Autodesk Inventor part; units mm, degrees
ref_plane "YZ Plane" through (0, 0, 0) normal (1, 0, 0) x (0, 1, 0)
ref_plane "XZ Plane" through (0, 0, 0) normal (0, 1, 0) x (-1, 0, 0)
ref_plane "XY Plane" through (0, 0, 0) normal (0, 0, 1) x (1, 0, 0)
sketch "스케치1" plane through (0, 0, 0) normal (1, 0, 0) x (0, 1, 0)
  circle A0 centre (0, 0) radius 55
  circle A1 centre (0, 0) radius 54
  dimension "d0" = 110
  dimension "d1" = 1
extrude "돌출1" add sketch "스케치1" along normal mid plane 36
sketch "스케치2" plane through (18, 0, 0) normal (1, 0, 0) x (0, 0, -1)
  circle A0 centre (0, 0) radius 55
  circle A1 centre (0, 0) radius 2
  dimension "d4" = 4
extrude "돌출2" add sketch "스케치2" against normal blind 1
sketch "스케치3" plane through (-18, 0, 0) normal (-1, 0, 0) x (0, 0, 1)
  circle A0 centre (0, 0) radius 2
  circle A1 centre (0, 0) radius 54
extrude "돌출3" add sketch "스케치3" against normal blind 1
sketch "스케치4" plane through (-18, 0, 0) normal (-1, 0, 0) x (0, 0, 1)
  circle A0 centre (0, 0) radius 14
  line L0 (0, 0) -> (14, 0)
  circle A1 centre (14, 0) radius 1.5
  dimension "d9" = 28
  dimension "d10" = 3
extrude "돌출4" cut sketch "스케치4" against normal blind 36 contours L0 A1 A0 | A0 A1 | A0 A1 L0 picked at (14.4441, -0.3905)
pattern_circular "원형 패턴1" count 4 over 360 about axis through (-18, 0, 0) along (1, 0, 0) of "돌출4"
fillet "모깎기1" radius 2 3 edges at (18, 38.8909, -38.8909) (18, -38.8909, 38.8909) (-18, -55, 0)
properties part number "바퀴"
CAD build for the part. Positions are in the model's coordinates, mm. A direction names the side the tool comes from. Round coordinates to 2 decimals unless told otherwise and drop trailing zeros. Order: outer loops, then holes, each group sorted by start corner. A loop starts at its lowest first (then second) coordinate and runs counter-clockwise, first axis right, second up. Notation, with made-up numbers: (25.5, 88) -> (48.5, 88) arc R11 cw to (48.5, 92) -> close; hole circle Ø9 at (-35, 29). An arc over 180 degrees is marked (long way). One line per question, with ' | ' between items.
Q1. Drop flat-ended pins along their axis: pin 1 (3 mm diameter, centred on x = 0, z = 5, fed in from -Y); pin 2 (3 mm diameter, centred on x = -12.5, z = -11, fed in from +Y); pin 3 (3.5 mm diameter, centred on y = 0, z = 0, fed in from -X); pin 4 (1.5 mm diameter, centred on x = -2, z = -28.5, fed in from -Y). Give the stop position or say it passes through.
Completed:
pin 1: stops at y = -54.89 | pin 2: stops at y = 54.17 | pin 3: passes through | pin 4: stops at y = -47.49
Q2. Two-plate mould, pull along X, no slides. Class faces 3 (the cylindrical face through (-17.507, -1.952, -0.434)), 4 (the cylindrical face through (0.238, -11.706, -52.716)), 5 (the flat face through (18, -1, 2)): released by +X, released by -X, zero draft, split by the parting line, or undercut.
Completed:
face 3: zero draft | face 4: undercut | face 5: released by +X
Q3. Slice it at A-A (z = 0). Give the number of separate pieces and of enclosed holes in the cut face, then the cut area to 3 significant figures.
Completed:
separate pieces: 6 | enclosed holes: 0 | area: 265 mm^2
Q4. Which spindle directions (+Z, -Z, +X, -X, +Y, -Y) get a long thin tool onto all of the face, cutting with end or side? Do faces 1 (the flat face through (17, 1, -11)), 2 (the flat face through (-18, 1, 11)). Say none if no direction does.
Completed:
face 1: none | face 2: +Z, -Z, -X, +Y, -Y
Q5. Slice it at B-B (x = -12). Write the cut outline in (y, z), then the cut area to 3 significant figures.
Completed:
outline: circle Ø110 at (0, 0); hole circle Ø108 at (0, 0) | area: 342 mm^2
Q6. Probe probe 1 along X at (y, z) = (26, -26); probe 2 along Z at (x, y) = (-17.75, -14); probe 3 along Z at (x, y) = (-1, 7). List the from-to ranges inside material, lowest first.
Completed:
probe 1: x = -18 to -17, 17 to 18 | probe 2: z = -52.12 to -1.5, 1.5 to 52.12 | probe 3: z = -54.55 to -53.54, 53.54 to 54.55
